```python
from build123d import *

# Parameters (mm, degrees)
F0_R     = 4.1
F0_R_2   = 2.725
F0_R_3   = 2.5
F0_R_4   = 3.6
F1_DEPTH = 10
F2_DEPTH = 6
F3_DEPTH = 4


# Not quite as in the source:
# - ends of sketch curves that miss each other by under 0.0002 mm in the source are joined


with BuildPart() as f1:
    # F0 (on Top) → F1 (new body)
    with BuildSketch(Plane.XY):
        with BuildLine():
            ThreePointArc((-70, -85.3407), (-69.01608381, -87.71608381), (-66.6407, -88.7))
            Line((-66.6407, -88.7), (66.64, -88.7))
            ThreePointArc((66.64, -88.7), (69.0158787848, -87.7158787848), (70, -85.34))
            Line((70, -85.34), (70, -67.5895))
            Line((70, -67.5895), (69.865948, -66.201885))
            Line((69.865948, -66.201885), (69.445962, -64.711612))
            Line((69.445962, -64.711612), (68.73318, -63.151071))
            Line((68.73318, -63.151071), (67.734412, -61.538447))
            Line((67.734412, -61.538447), (58.431324, -48.174831))
            ThreePointArc((58.431324, -48.174831), (58.1178035717, -47.5357835753), (58.01, -46.832182))
            Line((58.01, -46.832182), (58.01, -22.760348))
            ThreePointArc((58.01, -22.760348), (58.1179689174, -22.0562197272), (58.4319545741, -21.4167927032))
            Line((58.4319545741, -21.4167927032), (66.783489, -9.432068))
            Line((66.783489, -9.432068), (67.913719, -7.648339))
            Line((67.913719, -7.648339), (68.762828, -5.93532))
            Line((68.762828, -5.93532), (69.316332, -4.305329))
            Line((69.316332, -4.305329), (69.565046, -2.784029))
            Line((69.565046, -2.784029), (69.518711, -1.391715))
            Line((69.518711, -1.391715), (67.309142, 14.330181))
            Line((67.309142, 14.330181), (66.999212, 15.650057))
            Line((66.999212, 15.650057), (66.487155, 16.737863))
            Line((66.487155, 16.737863), (65.781814, 17.619854))
            Line((65.781814, 17.619854), (64.875084, 18.317561))
            Line((64.875084, 18.317561), (46.034788, 29.637953))
            ThreePointArc((46.034788, 29.637953), (45.2854954651, 30.3552438624), (44.917997067, 31.3252390094))
            Line((44.917997067, 31.3252390094), (40.093666, 65.65214))
            ThreePointArc((40.093666, 65.65214), (35.8358190199, 74.0012505725), (27.3375349502, 77.9529685197))
            ThreePointArc((27.3375349502, 77.9529685197), (26.1084756666, 78.4580664195), (25.3498539146, 79.5490309716))
            Line((25.3498539146, 79.5490309716), (24.828406, 81.117409))
            ThreePointArc((24.828406, 81.117409), (24.1173215696, 81.671357459), (24.355163875, 82.5408001437))
            ThreePointArc((24.355163875, 82.5408001437), (22.3679675258, 86.9125704183), (17.910791, 88.7))
            Line((17.910791, 88.7), (7.437437, 88.7))
            ThreePointArc((7.437437, 88.7), (6.5667217917, 88.5327402562), (5.8199517771, 88.0547702349))
            Line((5.8199517771, 88.0547702349), (3.5, 85.8536))
            ThreePointArc((3.5, 85.8536), (3.4660810953, 84.4733300764), (4.8463500657, 84.5072999404))
            Line((4.8463500657, 84.5072999404), (7.5, 84.5073))
            ThreePointArc((7.5, 84.5073), (11.5, 80.5073), (7.5, 76.5073))
            Line((7.5, 76.5073), (-7.5, 76.5073))
            ThreePointArc((-7.5, 76.5073), (-11.5, 80.5073), (-7.5, 84.5073))
            Line((-7.5, 84.5073), (-4.84635, 84.5073))
            ThreePointArc((-4.84635, 84.5073), (-3.4660810953, 84.4733300764), (-3.4999997219, 85.8536003068))
            Line((-3.4999997219, 85.8536003068), (-5.819951, 88.05477))
            ThreePointArc((-5.819951, 88.05477), (-6.5667214548, 88.5327401218), (-7.437437, 88.7))
            Line((-7.437437, 88.7), (-17.91079, 88.7))
            ThreePointArc((-17.91079, 88.7), (-22.3679665258, 86.9125704183), (-24.3551631887, 82.5408000085))
            ThreePointArc((-24.3551631887, 82.5408000085), (-24.1173207269, 81.6713569858), (-24.8284060254, 81.1174093435))
            Line((-24.8284060254, 81.1174093435), (-25.349853, 79.549031))
            ThreePointArc((-25.349853, 79.549031), (-26.1084746666, 78.4580664195), (-27.3375339495, 77.9529685125))
            ThreePointArc((-27.3375339495, 77.9529685125), (-35.8358186118, 74.001250966), (-40.0936657548, 65.6521401061))
            Line((-40.0936657548, 65.6521401061), (-44.917996, 31.325239))
            ThreePointArc((-44.917996, 31.325239), (-45.2854944651, 30.3552438624), (-46.0347868046, 29.6379526747))
            Line((-46.0347868046, 29.6379526747), (-64.875083, 18.317561))
            Line((-64.875083, 18.317561), (-65.764804, 17.636264))
            Line((-65.764804, 17.636264), (-66.464414, 16.773352))
            Line((-66.464414, 16.773352), (-66.99028, 15.673609))
            Line((-66.99028, 15.673609), (-67.30828, 14.330181))
            Line((-67.30828, 14.330181), (-69.517848, -1.391715))
            Line((-69.517848, -1.391715), (-69.564686, -2.784465))
            Line((-69.564686, -2.784465), (-69.316601, -4.307546))
            Line((-69.316601, -4.307546), (-68.763454, -5.938605))
            Line((-68.763454, -5.938605), (-67.915019, -7.650791))
            Line((-67.915019, -7.650791), (-66.786009, -9.432068))
            Line((-66.786009, -9.432068), (-58.427898, -21.419694))
            ThreePointArc((-58.427898, -21.419694), (-58.1136589115, -22.059327239), (-58.0056, -22.763742))
            Line((-58.0056, -22.763742), (-58.0056, -46.834916))
            ThreePointArc((-58.0056, -46.834916), (-58.1134934129, -47.5388038122), (-58.4272664273, -48.1780577023))
            Line((-58.4272664273, -48.1780577023), (-67.733176, -61.538447))
            Line((-67.733176, -61.538447), (-68.732469, -63.151034))
            Line((-68.732469, -63.151034), (-69.445644, -64.711573))
            Line((-69.445644, -64.711573), (-69.865872, -66.201869))
            Line((-69.865872, -66.201869), (-70, -67.5895))
            Line((-70, -67.5895), (-70, -85.3407))
        make_face()
        with Locations((-56.5, -75.18)):
            Circle(F0_R, mode=Mode.SUBTRACT)
        with Locations((56.5, -75.18)):
            Circle(F0_R, mode=Mode.SUBTRACT)
        with BuildLine():
            Line((19.8032, -63.6519), (-19.8032, -63.6519))
            ThreePointArc((-19.8032, -63.6519), (-31.1500010963, -58.9519010963), (-35.85, -47.6051))
            Line((-35.85, -47.6051), (-35.85, -21.9987))
            ThreePointArc((-35.85, -21.9987), (-31.1500010963, -10.6518989037), (-19.8032, -5.9519))
            Line((-19.8032, -5.9519), (19.8032, -5.9519))
            ThreePointArc((19.8032, -5.9519), (31.1500010963, -10.6518989037), (35.85, -21.9987))
            Line((35.85, -21.9987), (35.85, -47.6051))
            ThreePointArc((35.85, -47.6051), (31.1500010963, -58.9519010963), (19.8032, -63.6519))
        make_face(mode=Mode.SUBTRACT)
        with Locations((-56.5, 4.52)):
            Circle(F0_R, mode=Mode.SUBTRACT)
        with BuildLine():
            Line((-28.21, 12.7), (-28.21, 21.7))
            ThreePointArc((-28.21, 21.7), (-23.57, 26.34), (-18.93, 21.7))
            Line((-18.93, 21.7), (-18.93, 12.7))
            ThreePointArc((-18.93, 12.7), (-23.57, 8.06), (-28.21, 12.7))
        make_face(mode=Mode.SUBTRACT)
        with Locations((-33.8, 49.95)):
            Circle(F0_R_2, mode=Mode.SUBTRACT)
        with BuildLine():
            Line((-28.21, 59.84), (-28.21, 68.84))
            ThreePointArc((-28.21, 68.84), (-23.57, 73.48), (-18.93, 68.84))
            Line((-18.93, 68.84), (-18.93, 59.84))
            ThreePointArc((-18.93, 59.84), (-23.57, 55.2), (-28.21, 59.84))
        make_face(mode=Mode.SUBTRACT)
        with Locations((-17.9, 80.5073)):
            Circle(F0_R_2, mode=Mode.SUBTRACT)
        with BuildLine():
            Line((18.93, 12.7), (18.93, 21.7))
            ThreePointArc((18.93, 21.7), (23.57, 26.34), (28.21, 21.7))
            Line((28.21, 21.7), (28.21, 12.7))
            ThreePointArc((28.21, 12.7), (23.57, 8.06), (18.93, 12.7))
        make_face(mode=Mode.SUBTRACT)
        with BuildLine():
            Line((-12.5, 35.77), (-12.5, 45.77))
            ThreePointArc((-12.5, 45.77), (0, 58.27), (12.5, 45.77))
            Line((12.5, 45.77), (12.5, 35.77))
            ThreePointArc((12.5, 35.77), (0, 23.27), (-12.5, 35.77))
        make_face(mode=Mode.SUBTRACT)
        with Locations((56.5, 4.52)):
            Circle(F0_R, mode=Mode.SUBTRACT)
        with Locations((33.8, 49.95)):
            Circle(F0_R_2, mode=Mode.SUBTRACT)
        with BuildLine():
            Line((18.93, 59.84), (18.93, 68.84))
            ThreePointArc((18.93, 68.84), (23.57, 73.48), (28.21, 68.84))
            Line((28.21, 68.84), (28.21, 59.84))
            ThreePointArc((28.21, 59.84), (23.57, 55.2), (18.93, 59.84))
        make_face(mode=Mode.SUBTRACT)
        with Locations((17.9, 80.5073)):
            Circle(F0_R_2, mode=Mode.SUBTRACT)
        with Locations((-56.5, 4.52)):
            Circle(F0_R)
        with Locations((-56.5, 4.52)):
            Circle(F0_R_3, mode=Mode.SUBTRACT)
        with Locations((56.5, 4.52)):
            Circle(F0_R)
        with Locations((56.5, 4.52)):
            Circle(F0_R_3, mode=Mode.SUBTRACT)
        with Locations((56.5, -75.18)):
            Circle(F0_R)
        with Locations((56.5, -75.18)):
            Circle(F0_R_4, mode=Mode.SUBTRACT)
        with Locations((-56.5, -75.18)):
            Circle(F0_R)
        with Locations((-56.5, -75.18)):
            Circle(F0_R_4, mode=Mode.SUBTRACT)
    extrude(amount=F1_DEPTH)

    # F0 (on Top) → F2 (join)
    with BuildSketch(Plane.XY):
        with BuildLine():
            ThreePointArc((-18.93, 21.7), (-23.57, 26.34), (-28.21, 21.7))
            Line((-28.21, 21.7), (-28.21, 12.7))
            ThreePointArc((-28.21, 12.7), (-23.57, 8.06), (-18.93, 12.7))
            Line((-18.93, 12.7), (-18.93, 21.7))
        make_face()
        with BuildLine():
            Line((-26.11, 12.7), (-26.11, 21.7))
            ThreePointArc((-26.11, 21.7), (-23.57, 24.24), (-21.03, 21.7))
            Line((-21.03, 21.7), (-21.03, 12.7))
            ThreePointArc((-21.03, 12.7), (-23.57, 10.16), (-26.11, 12.7))
        make_face(mode=Mode.SUBTRACT)
        with BuildLine():
            ThreePointArc((-18.93, 68.84), (-23.57, 73.48), (-28.21, 68.84))
            Line((-28.21, 68.84), (-28.21, 59.84))
            ThreePointArc((-28.21, 59.84), (-23.57, 55.2), (-18.93, 59.84))
            Line((-18.93, 59.84), (-18.93, 68.84))
        make_face()
        with BuildLine():
            Line((-26.11, 59.84), (-26.11, 68.84))
            ThreePointArc((-26.11, 68.84), (-23.57, 71.38), (-21.03, 68.84))
            Line((-21.03, 68.84), (-21.03, 59.84))
            ThreePointArc((-21.03, 59.84), (-23.57, 57.3), (-26.11, 59.84))
        make_face(mode=Mode.SUBTRACT)
        with BuildLine():
            ThreePointArc((28.21, 68.84), (23.57, 73.48), (18.93, 68.84))
            Line((18.93, 68.84), (18.93, 59.84))
            ThreePointArc((18.93, 59.84), (23.57, 55.2), (28.21, 59.84))
            Line((28.21, 59.84), (28.21, 68.84))
        make_face()
        with BuildLine():
            Line((21.03, 59.84), (21.03, 68.84))
            ThreePointArc((21.03, 68.84), (23.57, 71.38), (26.11, 68.84))
            Line((26.11, 68.84), (26.11, 59.84))
            ThreePointArc((26.11, 59.84), (23.57, 57.3), (21.03, 59.84))
        make_face(mode=Mode.SUBTRACT)
        with BuildLine():
            ThreePointArc((28.21, 21.7), (23.57, 26.34), (18.93, 21.7))
            Line((18.93, 21.7), (18.93, 12.7))
            ThreePointArc((18.93, 12.7), (23.57, 8.06), (28.21, 12.7))
            Line((28.21, 12.7), (28.21, 21.7))
        make_face()
        with BuildLine():
            Line((21.03, 12.7), (21.03, 21.7))
            ThreePointArc((21.03, 21.7), (23.57, 24.24), (26.11, 21.7))
            Line((26.11, 21.7), (26.11, 12.7))
            ThreePointArc((26.11, 12.7), (23.57, 10.16), (21.03, 12.7))
        make_face(mode=Mode.SUBTRACT)
    extrude(amount=F2_DEPTH)

    # F0 (on Top) → F3 (cut, through all)
    with BuildSketch(Plane.XY):
        with Locations((-56.5, -75.18)):
            Circle(F0_R)
        with Locations((-56.5, -75.18)):
            Circle(F0_R_4, mode=Mode.SUBTRACT)
        with Locations((-56.5, 4.52)):
            Circle(F0_R)
        with Locations((-56.5, 4.52)):
            Circle(F0_R_3, mode=Mode.SUBTRACT)
        with Locations((56.5, 4.52)):
            Circle(F0_R)
        with Locations((56.5, 4.52)):
            Circle(F0_R_3, mode=Mode.SUBTRACT)
        with Locations((56.5, -75.18)):
            Circle(F0_R)
        with Locations((56.5, -75.18)):
            Circle(F0_R_4, mode=Mode.SUBTRACT)
    extrude(amount=F3_DEPTH, mode=Mode.SUBTRACT)


solid = f1.part
```
Here's how the part is built. I have some questions about the finished solid (model axes, mm). A direction names the side the tool comes from. Coordinates: 2 decimals unless noted, no trailing zeros. Order: outer loops, then holes, each group sorted by start corner. A loop starts at its lowest first (then second) coordinate and runs counter-clockwise, first axis right, second up. Notation, with made-up numbers: (84, 19.5) - (129, 19.5) arc R9 ccw to (129, 33.5) - close; hole circle Ø1 at (-36.75, -18). An arc over 180 degrees is marked (long way). One line per question, with ' | ' between items. Start each with the question number.
1. If we mould it in two halves opening along X, with no side actions, what happens to faces 1 (the cylindrical face through (53.478, -72.409, 1.972)), 2 (the flat face through (-58.006, -35, 5)), 3 (the flat face through (63.15, -54.95, 4.93))? For each: released by +X, released by -X, zero draft, split by the parting line, or undercut.
2. Please list where these lines run through material, in increasing order: line 1 along Y through (x, z) = (-17.9, 4.5); line 2 along X through (y, z) = (-30.5, 5); line 3 along X through (y, z) = (6, 9.5). Write a range as [from, to].
3. If we section it at B-B (z = 7.5): Give the number of separate pieces and of enclosed holes in the cut face, and give its area (3 significant figures).
4. I'm going to push flat-ended pins straight in: pin 1 Ø3 at (y, z) = (-34, 5) entering from +X; pin 2 Ø3 at (y, z) = (42.5, 3) entering from -X; pin 3 Ø1.2 at (y, z) = (19, 8) entering from +X; pin 4 Ø3 at (x, y) = (-56.5, 4.52) entering from +Z. Where does each tip first touch, or does it pass through?
5. If we section it at A-A (y = -75.18): Write out the boundary of the cut face in (x, z).
6. Which directions (+Z, -Z, +X, -X, +Y, -Y) give clear straight access to the entire face, cutting with the end or side of a thin tool? Please do faces 4 (the flat face through (-26.11, 17, 3)), 5 (the flat face through (-55.32, 24.06, 4.93)), 6 (the flat face through (18.93, 17, 8)), 7 (the cylindrical face through (-59.522, -72.409, 1.972)), 8 (the flat face through (-63.015, -54.765, 4.93)).
Model answer:
1) face 1: undercut | face 2: released by -X | face 3: released by +X
2) line 1: y = [-88.7, -63.65], [-5.95, 77.78], [83.23, 88.7] | line 2: x = [-58.01, -35.85], [35.85, 58.01] | line 3: x = [-68.48, -58.51], [-54.49, 54.49], [58.51, 68.48]
3) separate pieces: 1 | enclosed holes: 14 | area: 13,900 mm²
4) pin 1: stops at x = 58.01 | pin 2: stops at x = -43.56 | pin 3: stops at x = 64.74 | pin 4: passes through
5) outline: (-70, 0) - (-60.6, 0) - (-60.6, 4) - (-60.1, 4) - (-60.1, 10) - (-70, 10) - close; (-52.9, 4) - (-52.4, 4) - (-52.4, 0) - (52.4, 0) - (52.4, 4) - (52.9, 4) - (52.9, 10) - (-52.9, 10) - close; (60.1, 4) - (60.6, 4) - (60.6, 0) - (70, 0) - (70, 10) - (60.1, 10) - close
6) face 4: +Z, -Z | face 5: +Z, -Z, -X, +Y | face 6: +Z | face 7: -Z | face 8: +Z, -Z, -X
